Work out the finished part from the listing and answer in its coordinate system (mm). Round coordinates to 2 decimals unless told otherwise and drop trailing zeros. Loops run counter-clockwise (first coordinate to the right, second up) from the corner with the lowest first, then second, coordinate; pieces in that order, holes last.
from build123d import *

# Parameters (mm, degrees)
F0_W     = 40
F0_H     = 50
F0_H_2   = 150
F3_R     = 2
F2_R     = 40
F4_DEPTH = 23
F7_DEPTH = 25


with BuildPart() as f1:
    # F0 (on Front) → F1 (revolve)
    with BuildSketch(Plane.XZ):
        with Locations((-20, 25)):
            Rectangle(F0_W, F0_H)
        with Locations((-20, -75)):
            Rectangle(F0_W, F0_H_2)
    revolve(axis=Axis((0, 0, -53.9682246745), (0, 0, -1)))

    # F3
    f3_edges = [f1.edges().sort_by_distance(p)[0] for p in [
        (40, 0, 50),
    ]]
    fillet(f3_edges, radius=F3_R)

    # F2 (on face) → F4 (cut)
    with BuildSketch(Plane(origin=(0, 0, -150), x_dir=(1, 0, 0), z_dir=(0, 0, -1))):
        Circle(F2_R)
    extrude(amount=-F4_DEPTH, mode=Mode.SUBTRACT)

    # F5 (on Right) → F6 (revolve, cut)
    with BuildSketch(Plane.YZ):
        with BuildLine():
            ThreePointArc((-40, -121), (-41, -122), (-40, -123))
            Line((-40, -123), (-40, -122))
            Line((-40, -122), (-40, -121))
        make_face()
    revolve(axis=Axis((0, -40, -39.5), (0, 0, 1)), mode=Mode.SUBTRACT)

    # F7 (add): a face of the model
    f7_faces = [f1.faces().sort_by_distance(p)[0] for p in [
        (0, 0, -127),
    ]]
    extrude(f7_faces, amount=F7_DEPTH)


solid = f1.part
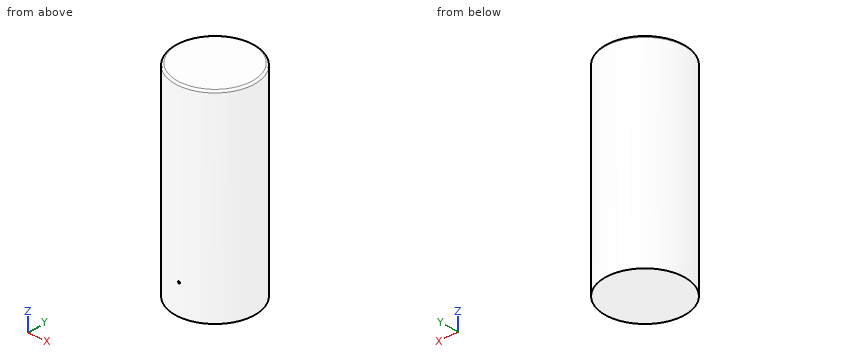
Item 1: Each of these flat-tipped pins is pushed along its axis until it touches: P1, Ø5, axis at x = -5.5, z = -59.5, coming from the -Y side; P2, Ø4, axis at y = -3.5, z = -34.5, coming from the -X side; P3, Ø1, axis at y = 19, z = -119, coming from the +X side. Where does it stop, or does it pass through?
Item 2: Straight lines are drawn through the part: line 1 (Y direction, x = 15.5, z = 29); line 2 (Y direction, x = -12, z = -36); line 3 (X direction, y = 29.5, z = -144). For each, find the intervals that lie inside material, in ascending order.
Item 3: Section A-A, the plane z = -62 is taken. Give the vertices of the cut face in (x, y).
Answer below:
1. P1: stops at y = -39.89
1. P2: stops at x = -39.97
1. P3: stops at x = 35.46
2. line 1: y = -36.87 to 36.87
2. line 2: y = -38.16 to 38.16
2. line 3: x = -27.01 to 27.01
3. outline: circle Ø80 at (0, 0)
